Geometry check sheet. Reference: the model listing, model coordinates, mm. Round coordinates to 2 decimals unless told otherwise and drop trailing zeros. Write item = value, one per line.
```python
from build123d import *

# Parameters (mm, degrees)
SKETCH1_W                  = 381
SKETCH1_H                  = 193.675
BOSS_EXTRUDE1_DEPTH        = 1.5
CUT_EXTRUDE1_DEPTH         = 214.72120018
CUT_EXTRUDE1_DEPTH_BACK    = 214.72120018
SKETCH2_W                  = 25.4
SKETCH2_H                  = 19.05
SKETCH2_W_2                = 22.225
SKETCH3_W                  = 19.05
SKETCH3_H                  = 12.7
BOSS_EXTRUDE2_DEPTH        = 3
FILLET1_R                  = 3.175
FILLET1_OF_MIRROR1_R       = 3.175
FILLET2_R                  = 1.5875
LPATTERN1_START            = -1.5
LPATTERN1_DEPTH            = 3
F_1_0MM_DOWEL_HOLE6_D      = 8
F_1_0MM_DOWEL_HOLE5_D      = 8
F_8_CLEARANCE_HOLE1_D      = 4.4958
F_1_0MM_DOWEL_HOLE1_D      = 4.8
F_1_0_4_8_DIAMETER_HOLE1_D = 4.8
LPATTERN2_COUNT            = 2
LPATTERN2_PITCH            = 50.8
LPATTERN2_COL_COUNT        = 2
LPATTERN2_COL_PITCH        = 50.8
MIRROR2_COPY_1_D           = 4.8
MIRROR2_COPY_2_D           = 4.8


# Read off the part's stored shape, not the designer's step: LPattern1
with BuildPart() as part:
    # Sketch1 → Boss-Extrude1 (new, symmetric)
    with BuildSketch(Plane.XY):
        Rectangle(SKETCH1_W, SKETCH1_H)
    extrude(amount=BOSS_EXTRUDE1_DEPTH, both=True)

    # Sketch2 → Cut-Extrude1 (cut, two sides: drawn at the far end of the back side and taken through both)
    with BuildSketch(Plane.XY.offset(1.5).offset(-CUT_EXTRUDE1_DEPTH_BACK)):
        with Locations((-177.8, 87.3125)):
            Rectangle(SKETCH2_W, SKETCH2_H)
        with Locations((80.9625, 87.3125)):
            Rectangle(SKETCH2_W_2, SKETCH2_H)
    extrude(amount=CUT_EXTRUDE1_DEPTH + CUT_EXTRUDE1_DEPTH_BACK, mode=Mode.SUBTRACT)

    # Sketch3 → Boss-Extrude2 (add)
    with BuildSketch(Plane.XY.offset(1.5)):
        with Locations((-200.025, -9.525)):
            Rectangle(SKETCH3_W, SKETCH3_H)
    boss_extrude2 = extrude(amount=-BOSS_EXTRUDE2_DEPTH)

    # Fillet1
    fillet1_edges = [part.edges().sort_by_distance(p)[0] for p in [
        (-209.55, -3.175, 0),
        (-209.55, -15.875, 0),
    ]]
    fillet(fillet1_edges, radius=FILLET1_R)

    # Mirror1: Boss-Extrude2 across plane
    add(boss_extrude2.mirror(Plane(origin=(0, 0, 0), x_dir=(0, 0, 1), z_dir=(1, 0, 0))))

    # Fillet1 of Mirror1
    fillet1_of_mirror1_edges = [part.edges().sort_by_distance(p)[0] for p in [
        (209.55, -3.175, 0),
        (209.55, -15.875, 0),
    ]]
    fillet(fillet1_of_mirror1_edges, radius=FILLET1_OF_MIRROR1_R)

    # Fillet2
    fillet2_edges = [part.edges().sort_by_distance(p)[0] for p in [
        (-190.5, -15.875, 0),
        (-190.5, -3.175, 0),
        (190.5, -15.875, 0),
        (190.5, -3.175, 0),
    ]]
    fillet(fillet2_edges, radius=FILLET2_R)

    # LPattern1 outline → LPattern1 (add)
    with BuildSketch(Plane.XY.offset(LPATTERN1_START)):
        with BuildLine():
            ThreePointArc((-206.375, 47.625), (-208.62006403, 46.69506403), (-209.55, 44.45))
            Line((-209.55, 44.45), (-209.55, 38.1))
            ThreePointArc((-209.55, 38.1), (-208.62006403, 35.85493597), (-206.375, 34.925))
            Line((-206.375, 34.925), (-192.0875, 34.925))
            ThreePointArc((-192.0875, 34.925), (-190.964967985, 34.460032015), (-190.5, 33.3375))
            Line((-190.5, 33.3375), (-190.5, 49.2125))
            ThreePointArc((-190.5, 49.2125), (-190.964967985, 48.089967985), (-192.0875, 47.625))
            Line((-192.0875, 47.625), (-206.375, 47.625))
        make_face()
        with BuildLine():
            ThreePointArc((-206.375, -53.975), (-208.62006403, -54.90493597), (-209.55, -57.15))
            Line((-209.55, -57.15), (-209.55, -63.5))
            ThreePointArc((-209.55, -63.5), (-208.62006403, -65.74506403), (-206.375, -66.675))
            Line((-206.375, -66.675), (-192.0875, -66.675))
            ThreePointArc((-192.0875, -66.675), (-190.964967985, -67.139967985), (-190.5, -68.2625))
            Line((-190.5, -68.2625), (-190.5, -52.3875))
            ThreePointArc((-190.5, -52.3875), (-190.964967985, -53.510032015), (-192.0875, -53.975))
            Line((-192.0875, -53.975), (-206.375, -53.975))
        make_face()
        with BuildLine():
            Line((209.55, 38.1), (209.55, 44.45))
            ThreePointArc((209.55, 44.45), (208.62006403, 46.69506403), (206.375, 47.625))
            Line((206.375, 47.625), (192.0875, 47.625))
            ThreePointArc((192.0875, 47.625), (190.964967985, 48.089967985), (190.5, 49.2125))
            Line((190.5, 49.2125), (190.5, 33.3375))
            ThreePointArc((190.5, 33.3375), (190.964967985, 34.460032015), (192.0875, 34.925))
            Line((192.0875, 34.925), (206.375, 34.925))
            ThreePointArc((206.375, 34.925), (208.62006403, 35.85493597), (209.55, 38.1))
        make_face()
        with BuildLine():
            Line((209.55, -63.5), (209.55, -57.15))
            ThreePointArc((209.55, -57.15), (208.62006403, -54.90493597), (206.375, -53.975))
            Line((206.375, -53.975), (192.0875, -53.975))
            ThreePointArc((192.0875, -53.975), (190.964967985, -53.510032015), (190.5, -52.3875))
            Line((190.5, -52.3875), (190.5, -68.2625))
            ThreePointArc((190.5, -68.2625), (190.964967985, -67.139967985), (192.0875, -66.675))
            Line((192.0875, -66.675), (206.375, -66.675))
            ThreePointArc((206.375, -66.675), (208.62006403, -65.74506403), (209.55, -63.5))
        make_face()
    extrude(amount=LPATTERN1_DEPTH)

    # Ø1.0mm Dowel Hole6 (through all)
    with Locations(Plane.XY.offset(1.5)):
        with Locations((114.080868605, -1.328387664)):
            Hole(F_1_0MM_DOWEL_HOLE6_D / 2)

    # Ø1.0mm Dowel Hole5 (through all)
    with Locations(Plane.XY.offset(1.5)):
        with Locations((62.931618599, -25.649221104)):
            Hole(F_1_0MM_DOWEL_HOLE5_D / 2)

    # #8 Clearance Hole1 (through all)
    with Locations(Plane(origin=(0, 0, -1.5), x_dir=(-1, 0, 0), z_dir=(0, 0, -1))):
        with Locations((3.488631395, 16.97194676), (-28.261368605, 16.97194676), (-28.261368605, -14.77805324), (3.488631395, -14.77805324), (-56.930868605, -87.847137664), (-114.080868605, -87.847137664), (-171.230868605, -87.847137664), (-165.723368605, 27.246612336), (-181.598368605, 27.246612336), (-181.598368605, -31.490887664), (-165.723368605, -31.490887664), (176.53, 66.736172691), (-97.1296, 88.08565122), (-141.5796, 62.422431754), (165.1, -71.4375)):
            Hole(F_8_CLEARANCE_HOLE1_D / 2)

    # Ø1.0mm Dowel Hole1 (through all)
    with Locations(Plane.XY.offset(1.5)):
        with Locations((-158.944770876, 59.513399002), (-48.646302539, 40.064803103), (-103.795536708, 49.789101052), (-41.555686717, 38.814536224), (13.593547451, 29.090238275), (68.74278162, 19.365940325), (67.618368605, 10.356435791), (67.618368605, -5.643564209), (155.263089531, -18.7625), (155.263089531, 93.2375), (168.480868605, -71.388387664), (168.480868605, -39.388387664)):
            Hole(F_1_0MM_DOWEL_HOLE1_D / 2)

    # Ø1.0 (4.8) Diameter Hole1 (through all)
    with Locations(Plane.XY.offset(1.5)):
        with Locations((196.65, -9.525)):
            f_1_0_4_8_diameter_hole1 = Hole(F_1_0_4_8_DIAMETER_HOLE1_D / 2)

    # LPattern2: Ø1.0 (4.8) Diameter Hole1 ×2
    with Locations(*[(0, i * LPATTERN2_PITCH, 0) for i in range(1, LPATTERN2_COUNT)]):
        add(f_1_0_4_8_diameter_hole1, mode=Mode.SUBTRACT)

    # LPattern2 col: Ø1.0 (4.8) Diameter Hole1 ×2
    with Locations(*[(0, -i * LPATTERN2_COL_PITCH, 0) for i in range(1, LPATTERN2_COL_COUNT)]):
        add(f_1_0_4_8_diameter_hole1, mode=Mode.SUBTRACT)

    # Mirror2: Ø1.0 (4.8) Diameter Hole1 across plane
    add(f_1_0_4_8_diameter_hole1.mirror(Plane(origin=(0, 0, 0), x_dir=(0, 0, 1), z_dir=(1, 0, 0))), mode=Mode.SUBTRACT)

    # Mirror2 copy 1 (through all)
    with Locations(Plane(origin=(0, 50.8, 1.5), x_dir=(-1, 0, 0), z_dir=(0, 0, 1))):
        with Locations((196.65, 9.525)):
            Hole(MIRROR2_COPY_1_D / 2)

    # Mirror2 copy 2 (through all)
    with Locations(Plane(origin=(0, -50.8, 1.5), x_dir=(-1, 0, 0), z_dir=(0, 0, 1))):
        with Locations((196.65, 9.525)):
            Hole(MIRROR2_COPY_2_D / 2)


solid = part.part
```
(1) Scan lines: L1, parallel to Y at x = 196.65, z = 0.8 (3 decimals); L2, parallel to X at y = 84, z = -0.7 (3 decimals); L3, parallel to X at y = 15, z = -1.3. Record each from-to range of solid material in increasing order. Write a range as [from, to].
Answers follow:
L1 = [-66.675, -62.725], [-57.925, -53.975], [-15.875, -11.925], [-7.125, -3.175], [34.925, 38.875], [43.675, 47.625]
L2 = [-165.1, 69.85], [92.075, 190.5]
L3 = [-190.5, -4.57], [-2.41, 27.18], [29.34, 190.5]
(2) Mould release check, pull along X, two halves, no side actions. Record for faces 1 (the flat face through (-3, 1, -1.5)), 2 (the cylindrical face through (65.88, -22.946, -0.021)): pulls with the +X half, pulls with the -X half, needs draft (parallel to the pull), parting line crosses it, or undercut.
Answers follow:
face_1 = needs draft
face_2 = undercut
(3) Section check A-A (z = 1). State how many separate pieces and enclosed holes the cut face has, then the cut area to 3 significant figures.
Answers follow:
separate_pieces = 1
enclosed_holes = 35
area = 73,700 mm²
(4) Gauge pin test, flat ends, axial feed: pin 1 (0.9 mm diameter, centred on y = 24, z = 0, fed in from -X); pin 2 (0.9 mm diameter, centred on x = -200, z = -0.5, fed in from +Y) (3 decimals); pin 3 (0.9 mm diameter, centred on x = 199, z = 0, fed in from -Y) (3 decimals). Record the tip position at first contact, or that the pin passes through.
Answers follow:
pin_1 = -190.5
pin_2 = 47.625
pin_3 = -66.675
